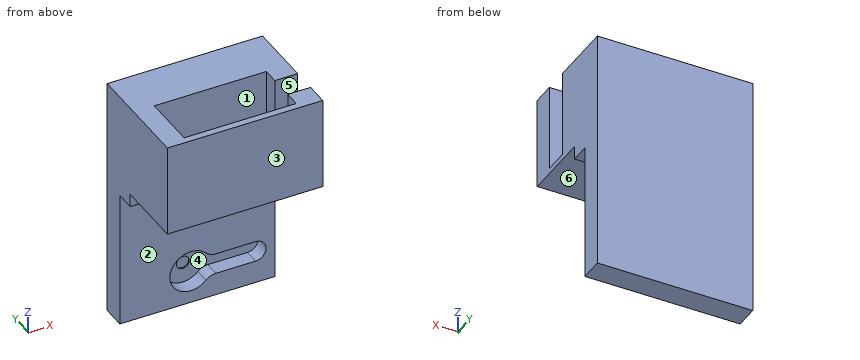
```python
from build123d import *

# Parameters (mm, degrees)
BOSS_EXTRUDE1_DEPTH = 31.5
CUT_EXTRUDE1_DEPTH  = 26.7
SKETCH3_W           = 56.2
SKETCH3_H           = 25.2
BOSS_EXTRUDE2_DEPTH = 2
SKETCH5_W           = 56.2
SKETCH5_H           = 20
BOSS_EXTRUDE4_DEPTH = 7
SKETCH6_W           = 56.2
SKETCH6_H           = 60
BOSS_EXTRUDE5_DEPTH = 8.5
CUT_EXTRUDE2_DEPTH  = 5.5
SKETCH11_R          = 2.32571443
CUT_EXTRUDE3_DEPTH  = 0.5
SKETCH12_W          = 56.2
SKETCH12_H          = 7
BOSS_EXTRUDE8_DEPTH = 18.321145389
SKETCH18_W          = 56.2
SKETCH18_H          = 8.5
BOSS_EXTRUDE9_DEPTH = 28.321145389
FILLET5_R           = 5


with BuildPart() as part:
    # Sketch1 → Boss-Extrude1 (new body)
    with BuildSketch(Plane.XY):
        Polygon((-3.384140796, -1.386438558), (-3.384140796, 23.813561442), (52.815859204, 23.813561442), (52.815859204, 15.563561442), (44.565859204, 15.563561442), (44.565859204, 6.863561442), (52.815859204, 6.863561442), (52.815859204, -1.386438558), align=None)
    extrude(amount=BOSS_EXTRUDE1_DEPTH)

    # Sketch2 → Cut-Extrude1 (cut)
    with BuildSketch(Plane.XY.offset(31.5)):
        Polygon((4.015859204, 21.313561442), (44.565859204, 21.313561442), (44.565859204, 15.563561442), (44.565859204, 6.863561442), (44.565859204, 1.113561442), (4.015859204, 1.113561442), align=None)
    extrude(amount=-CUT_EXTRUDE1_DEPTH, mode=Mode.SUBTRACT)

    # Sketch3 → Boss-Extrude2 (add)
    with BuildSketch(Plane(origin=(0, 0, 0), x_dir=(-1, 0, 0), z_dir=(0, 0, -1))):
        with Locations((-24.715859204, 11.213561442)):
            Rectangle(SKETCH3_W, SKETCH3_H)
    extrude(amount=BOSS_EXTRUDE2_DEPTH)

    # Sketch5 → Boss-Extrude4 (add)
    with BuildSketch(Plane(origin=(0, 23.813561442, 0), x_dir=(1, 0, 0), z_dir=(0, 1, 0))):
        with Locations((24.715859204, -3.178854611)):
            Rectangle(SKETCH5_W, SKETCH5_H)
    extrude(amount=BOSS_EXTRUDE4_DEPTH)

    # Sketch6 → Boss-Extrude5 (add)
    with BuildSketch(Plane(origin=(0, 30.813561442, 0), x_dir=(1, 0, 0), z_dir=(0, 1, 0))):
        with Locations((24.715859204, 26.821145389)):
            Rectangle(SKETCH6_W, SKETCH6_H)
    extrude(amount=BOSS_EXTRUDE5_DEPTH)

    # Sketch10 → Cut-Extrude2 (cut)
    with BuildSketch(Plane.XZ.offset(-30.813561442)):
        with BuildLine():
            Line((28.922300324, -40.947940044), (45.722300324, -40.947940044))
            ThreePointArc((45.722300324, -40.947940044), (49.522300324, -44.747940044), (45.722300324, -48.547940044))
            Line((45.722300324, -48.547940044), (28.922300324, -48.547940044))
            ThreePointArc((28.922300324, -48.547940044), (14.740507255, -44.747940044), (28.922300324, -40.947940044))
        make_face()
    extrude(amount=-CUT_EXTRUDE2_DEPTH, mode=Mode.SUBTRACT)

    # Sketch11 → Cut-Extrude3 (cut)
    with BuildSketch(Plane.XZ.offset(-36.313561442)):
        with Locations(Location((22.340507255, -44.747940044, 0), (0, 0, 270))):
            Circle(SKETCH11_R)
    extrude(amount=-CUT_EXTRUDE3_DEPTH, mode=Mode.SUBTRACT)

    # Sketch12 → Boss-Extrude8 (add)
    with BuildSketch(Plane.XY.offset(13.178854611)):
        with Locations((24.715859204, 27.313561442)):
            Rectangle(SKETCH12_W, SKETCH12_H)
    extrude(amount=BOSS_EXTRUDE8_DEPTH)

    # Sketch18 → Boss-Extrude9 (add)
    with BuildSketch(Plane.XY.offset(3.178854611)):
        with Locations((24.715859204, 35.063561442)):
            Rectangle(SKETCH18_W, SKETCH18_H)
    extrude(amount=BOSS_EXTRUDE9_DEPTH)

    # Fillet5
    fillet5_edges = [part.edges().sort_by_distance(p)[0] for p in [
        (28.922300324, 33.563561442, -48.547940044),
        (28.922300324, 33.563561442, -40.947940044),
    ]]
    fillet(fillet5_edges, radius=FILLET5_R)


solid = part.part
```
Can you work these out from the model? Positions are in its coordinate system, mm. Face numbers are marked on the shaded views. A direction names the side the tool comes from. Coordinates: 2 decimals unless noted, no trailing zeros. Order: outer loops, then holes, each group sorted by start corner. A loop starts at its lowest first (then second) coordinate and runs counter-clockwise, first axis right, second up.
1. If we section it at D-D (z = 7): Please give me the cut outline in (x, y).
2. For the marked faces 1, 2 and 3, which set-ups out of +Z, -Z, +X, -X, +Y, -Y let a thin tool reach every point of the face, with its end or its side?
3. If we section it at B-B (x = 39): Please give me the cut outline in (y, z).
4. If we section it at A-A (y = 33): Please give me the cut outline in (x, z), then the cut area to 3 significant figures.
5. If we section it at C-C (y = 18): Please give me the cut outline in (x, z), then the cut area to 3 significant figures.
6. I'm going to push flat-ended pins straight in: pin 1 (12 mm diameter, centred on x = 35, z = -14, fed in from -Y); pin 2 (4 mm diameter, centred on x = 34.5, z = -4.5, fed in from -Y); pin 3 (4 mm diameter, centred on x = 50.5, y = 13, fed in from +Z). Where does each tip first touch, or does it pass through?
7. Thinking about a two-plate mould opening in Y: for the marked faces 4, 5 and 6, which applies, +Y half, -Y half, draft (parallel to the pull), parting line (faces both ways), or undercut?
8. I need wall thicknesses on line 1 (Y direction, x = 49.5, z = 21.5); line 2 (Y direction, x = 40, z = 5); line 3 (X direction, y = 20, z = 9.5). Which ranges of each line are inside material? Lowest first, please.
Entries:
1. outline: (-3.38, -1.39) - (52.82, -1.39) - (52.82, 6.86) - (44.57, 6.86) - (44.57, 1.11) - (4.02, 1.11) - (4.02, 21.31) - (44.57, 21.31) - (44.57, 15.56) - (52.82, 15.56) - (52.82, 39.31) - (-3.38, 39.31) - close
2. face 1: +Z
2. face 2: -Z, +X, -X, -Y
2. face 3: +Z, -Z, +X, -X, -Y
3. outline: (-1.39, -2) - (23.81, -2) - (23.81, -6.82) - (30.81, -6.82) - (30.81, -40.95) - (36.31, -40.95) - (36.31, -48.55) - (30.81, -48.55) - (30.81, -56.82) - (39.31, -56.82) - (39.31, 31.5) - (21.31, 31.5) - (21.31, 4.8) - (1.11, 4.8) - (1.11, 31.5) - (-1.39, 31.5) - close
4. outline: (-3.38, -56.82) - (52.82, -56.82) - (52.82, 31.5) - (-3.38, 31.5) - close; hole (27.78, -50.06) arc R5 cw to (31.36, -48.55) - (45.72, -48.55) arc R3.8 ccw to (45.72, -40.95) - (31.36, -40.95) arc R5 cw to (27.78, -39.44) arc R7.6 ccw (long way) to start
4. area: 4,640 mm2
5. outline: (-3.38, -2) - (52.82, -2) - (52.82, 31.5) - (44.57, 31.5) - (44.57, 4.8) - (4.02, 4.8) - (4.02, 31.5) - (-3.38, 31.5) - close
5. area: 800 mm2
6. pin 1: stops at y = 30.81
6. pin 2: stops at y = 23.81
6. pin 3: stops at z = 0
7. face 4: -Y half
7. face 5: undercut
7. face 6: draft
8. line 1: y = -1.39 to 6.86, 15.56 to 39.31
8. line 2: y = -1.39 to 1.11, 21.31 to 39.31
8. line 3: x = -3.38 to 4.02, 44.57 to 52.82
